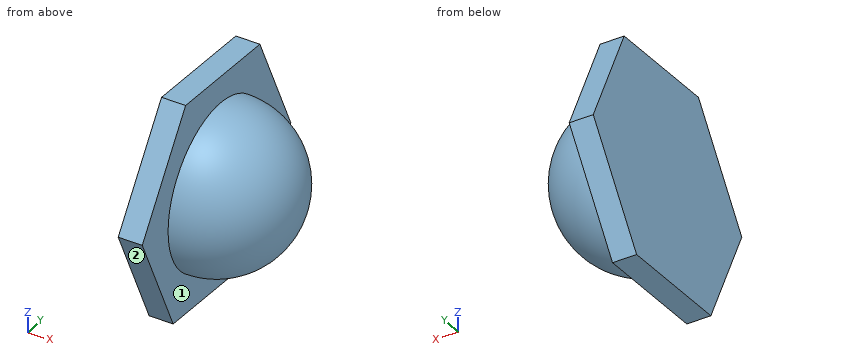
from build123d import *

# Parameters (mm, degrees)
F1_ANGLE = 180
F3_DEPTH = 2.2


with BuildPart() as f1:
    # F0 (on Right) → F1 (revolve)
    with BuildSketch(Plane.YZ):
        with BuildLine():
            ThreePointArc((0, -7.5), (7.5, 0), (0, 7.5))
            Line((0, 7.5), (0, -7.5))
        make_face()
    revolve(axis=Axis((0, 0, 0), (0, 0, -1)), revolution_arc=F1_ANGLE)

    # F2 (on Right) → F3 (join)
    with BuildSketch(Plane.YZ):
        Polygon((-4.788409, 10.514467), (-11.5, 1.110349), (-6.711591, -9.404118), (4.788409, -10.514467), (11.5, -1.110349), (6.711591, 9.404118), align=None)
    extrude(amount=-F3_DEPTH)


solid = f1.part
Can you work these out from the model? Positions are in its coordinate system, mm. Face numbers are marked on the shaded views. A direction names the side the tool comes from. Round coordinates to 2 decimals unless told otherwise and drop trailing zeros. Order: outer loops, then holes, each group sorted by start corner. A loop starts at its lowest first (then second) coordinate and runs counter-clockwise, first axis right, second up. Notation, with made-up numbers: M 39,15 L 62,15 A16 ccw 62,23 Z; hole C -18.5,31.25 d6. An arc over 180 degrees is marked long. Use a Markdown table: item, result.
1) I'm going to push flat-ended pins straight in: P1, Ø1.5, axis at y = -5, z = -4, coming from the +X side; P2, Ø3, axis at y = -2, z = 1, coming from the +X side; P3, Ø3, axis at y = -2, z = -5.5, coming from the +X side. Where does each tip first touch, or does it pass through?
Geometry says:
| item | result |
|---|---|
| P1 | stops at x = 4.93 |
| P2 | stops at x = 7.46 |
| P3 | stops at x = 6.11 |
2) Imagine slicing it at A-A (z = 3.25). List the corners of the cut face in (x, y) for me.
Geometry says:
| item | result |
|---|---|
| outline | M -2.2,-9.97 L 0,-9.97 L 0,-6.76 A6.76 ccw 0,6.76 L 0,9.51 L -2.2,9.51 Z |
3) Imagine slicing it at C-C (y = 10.25). List the corners of the cut face in (x, z) for me, then the cut area to 3 significant figures.
Geometry says:
| item | result |
|---|---|
| outline | M -2.2,-2.86 L 0,-2.86 L 0,1.63 L -2.2,1.63 Z |
| area | 9.89 mm² |
4) Imagine slicing it at B-B (x = -1). List the corners of the cut face in (y, z) for me, then the cut area to 3 significant figures.
Geometry says:
| item | result |
|---|---|
| outline | M -11.5,1.11 L -6.71,-9.4 L 4.79,-10.51 L 11.5,-1.11 L 6.71,9.4 L -4.79,10.51 Z |
| area | 347 mm² |
5) Imagine slicing it at D-D (x = 2). List the corners of the cut face in (y, z) for me.
Geometry says:
| item | result |
|---|---|
| outline | C 0,0 d14.46 |
6) On a 3-axis mill with a long thin cutter (end or side, diameter ignored), from which of +Z, -Z, +X, -X, +Y, -Y can I reach the whole of each face in a straight line? I mean the marked faces 1 and 2. Say none if no direction works.
Geometry says:
| item | result |
|---|---|
| face 1 | +X |
| face 2 | -Z, +X, -X, -Y |
7) If I drill on line 1 along X through (y, z) = (-8, 2.75); line 2 along Y through (x, z) = (5.5, -0.75); line 3 along Y through (x, z) = (4, 0), over which ranges is the centre line in solid material (lowest first)?
Geometry says:
| item | result |
|---|---|
| line 1 | x = -2.2 to 0 |
| line 2 | y = -5.04 to 5.04 |
| line 3 | y = -6.34 to 6.34 |
